Verification items for the finished model (mm, model axes). A direction names the side the tool comes from. Give positions to 0.01 mm unless a question says otherwise; leave off trailing zeros. Loops run counter-clockwise (first coordinate to the right, second up) from the corner with the lowest first, then second, coordinate; pieces in that order, holes last. Notation, with made-up numbers: M 66.5,69 L 89.5,69 A26 ccw 89.5,101 Z; hole C -27,-32 d10. An arc over 180 degrees is marked long. Write each question's results on one line, items separated by ' | '. Start each with the question number.
Autodesk Inventor part; units mm, degrees
ref_plane "YZ Plane" through (0, 0, 0) normal (1, 0, 0) x (0, 1, 0)
ref_plane "XZ Plane" through (0, 0, 0) normal (0, 1, 0) x (-1, 0, 0)
ref_plane "XY Plane" through (0, 0, 0) normal (0, 0, 1) x (1, 0, 0)
sketch "Sketch2" plane through (0, 0, 0) normal (0, 1, 0) x (-1, 0, 0)
  line L0 (35.4299, 28.2779) -> (35.4299, 34.5151)
  line L1 (35.4299, 51.0151) -> (35.4299, 60.0151)
  line L2 (47.4299, 49.0151) -> (37.4299, 49.0151)
  line L3 (20.9299, 49.0151) -> (12.9299, 49.0151)
  line L4 (22.9299, 55.7744) -> (22.9299, 51.0151)
  line L5 (22.9299, 34.5151) -> (22.9299, 26.5151)
  line L6 (12.9299, 36.5151) -> (20.9299, 36.5151)
  line L7 (37.4299, 36.5151) -> (47.4299, 36.5151)
  line L8 (12.9299, 38.5151) -> (14.9299, 38.5151)
  line L9 (14.9299, 38.5151) -> (14.9299, 40.0151)
  line L10 (14.9299, 40.0151) -> (12.9299, 40.0151)
  line L11 (12.9299, 42.0151) -> (14.9299, 42.0151)
  line L12 (14.9299, 42.0151) -> (14.9299, 43.5151)
  line L13 (14.9299, 43.5151) -> (12.9299, 43.5151)
  line L14 (12.9299, 45.5151) -> (14.9299, 45.5151)
  line L15 (14.9299, 45.5151) -> (14.9299, 47.0151)
  line L16 (14.9299, 47.0151) -> (12.9299, 47.0151)
  line L17 (12.9299, 49.0151) -> (12.9299, 47.0151)
  line L18 (12.9299, 45.5151) -> (12.9299, 43.5151)
  line L19 (12.9299, 42.0151) -> (12.9299, 40.0151)
  line L20 (12.9299, 38.5151) -> (12.9299, 36.5151)
  line L21 (33.4299, 27.5151) -> (33.4299, 25.5151)
  line L22 (31.9299, 25.5151) -> (31.9299, 27.5151)
  line L23 (29.9299, 27.5151) -> (29.9299, 25.5151)
  line L24 (28.4299, 25.5151) -> (28.4299, 27.5151)
  line L25 (26.4299, 27.5151) -> (26.4299, 25.5151)
  line L26 (24.9299, 25.5151) -> (24.9299, 27.5151)
  line L27 (47.4299, 47.0151) -> (45.4299, 47.0151)
  line L28 (47.4299, 45.5151) -> (45.4299, 45.5151)
  line L29 (47.4299, 43.5151) -> (45.4299, 43.5151)
  line L30 (47.4299, 42.0151) -> (45.4299, 42.0151)
  line L31 (47.4299, 40.0151) -> (45.4299, 40.0151)
  line L32 (47.4299, 38.5151) -> (45.4299, 38.5151)
  line L33 (45.4299, 38.5151) -> (45.4299, 40.0151)
  line L34 (45.4299, 42.0151) -> (45.4299, 43.5151)
  line L35 (45.4299, 45.5151) -> (45.4299, 47.0151)
  line L36 (47.4299, 36.5151) -> (47.4299, 38.5151)
  line L37 (47.4299, 40.0151) -> (47.4299, 42.0151)
  line L38 (47.4299, 43.5151) -> (47.4299, 45.5151)
  line L39 (47.4299, 47.0151) -> (47.4299, 49.0151)
  line L40 (33.4299, 60.0151) -> (33.4299, 58.0151)
  line L41 (31.9299, 60.0151) -> (31.9299, 58.0151)
  line L42 (29.9299, 60.0151) -> (29.9299, 58.0151)
  line L43 (28.4299, 60.0151) -> (28.4299, 58.0151)
  line L44 (26.4299, 60.0151) -> (26.4299, 58.0151)
  line L45 (24.9299, 60.0151) -> (24.9299, 58.0151)
  arc A0 (35.4299, 51.0151) -> (37.4299, 49.0151) centre (37.4299, 51.0151) ccw
  arc A1 (37.4299, 36.5151) -> (35.4299, 34.5151) centre (37.4299, 34.5151) ccw
  arc A2 (22.9299, 34.5151) -> (20.9299, 36.5151) centre (20.9299, 34.5151) ccw
  arc A3 (20.9299, 49.0151) -> (22.9299, 51.0151) centre (20.9299, 51.0151) ccw
  line L46 (35.4299, 28.2779) -> (35.4299, 25.5151)
  line L47 (22.9299, 26.5151) -> (22.9299, 25.5151)
  line L48 (35.4299, 25.5151) -> (33.4299, 25.5151)
  line L49 (31.9299, 25.5151) -> (29.9299, 25.5151)
  line L50 (28.4299, 25.5151) -> (26.4299, 25.5151)
  line L51 (24.9299, 25.5151) -> (22.9299, 25.5151)
  line L52 (24.9299, 27.5151) -> (26.4299, 27.5151)
  line L53 (28.4299, 27.5151) -> (29.9299, 27.5151)
  line L54 (31.9299, 27.5151) -> (33.4299, 27.5151)
  line L55 (22.9299, 55.7744) -> (22.9299, 60.0151)
  line L56 (35.4299, 60.0151) -> (33.4299, 60.0151)
  line L57 (31.9299, 60.0151) -> (29.9299, 60.0151)
  line L58 (28.4299, 60.0151) -> (26.4299, 60.0151)
  line L59 (24.9299, 60.0151) -> (22.9299, 60.0151)
  line L60 (24.9299, 58.0151) -> (26.4299, 58.0151)
  line L61 (28.4299, 58.0151) -> (29.9299, 58.0151)
  line L62 (31.9299, 58.0151) -> (33.4299, 58.0151)
  circle A4 centre (29.1799, 42.7651) radius 5.5
  point P0 (0, 0)
  point P1 (35.4299, 36.5151)
  point P2 (35.4299, 49.0151)
  point P3 (22.9299, 49.0151)
  point P4 (22.9299, 36.5151)
  dimension "d25" = 1.5
  dimension "d26" = 1.5
  dimension "d27" = 1.5
  dimension "d28" = 2
  dimension "d29" = 2
  dimension "d30" = 2
  dimension "d31" = 2
  dimension "d43" = 2
  dimension "d44" = 2
  dimension "d45" = 2
  dimension "d46" = 2
  dimension "d47" = 2
  dimension "d48" = 2
  dimension "d49" = 2
  dimension "d50" = 2
  dimension "d51" = 2
  dimension "d52" = 2
  dimension "d53" = 2
  dimension "d60" = 2
  dimension "d61" = 1.5
  dimension "d62" = 1.5
  dimension "d63" = 1.5
  dimension "d64" = 1.5
  dimension "d65" = 1.5
  dimension "d66" = 1.5
  dimension "d67" = 1.5
  dimension "d68" = 1.5
  dimension "d69" = 1.5
  dimension "d70" = 2
  dimension "d71" = 2
  dimension "d72" = 2
  dimension "d74" = 2
  dimension "d75" = 2
  dimension "d76" = 2
  dimension "d77" = 2
  dimension "d78" = 2
  dimension "d79" = 2
  dimension "d80" = 2
  dimension "d81" = 11
  dimension "d82" = 11
  dimension "d83" = 11
  dimension "d84" = 11
  dimension "d85" = 2
  dimension "d86" = 2
  dimension "d87" = 2
  dimension "d88" = 2
  dimension "d89" = 10
  dimension "d90" = 10
  dimension "d91" = 12
  dimension "d92" = 12
  dimension "d97" = 2
  dimension "d98" = 2
  dimension "d99" = 2
  dimension "d100" = 8
  dimension "d102" = 2
  dimension "d105" = 6.25
  dimension "d106" = 6.25
  dimension "d109" = 2
  dimension "d110" = 0
  dimension "d111" = 2
  dimension "d112" = 0
  dimension "d113" = 2
extrude "Extrusion3" add sketch "Sketch2" along normal blind 1.524
properties part number "cross"
1. Set-up check for faces 4 (the face through (-14, 1, 38.515)), 5 (the face through (-46, 1, 38.515)), 6 (the face through (-26, 1, 27.515)), 7 (the face through (-31.93, 1, 59)): record each of +Z, -Z, +X, -X, +Y, -Y from which the full face is reachable in a straight line by a thin tool's end or side.
2. Release check for a two-part mould opening along Z. For faces 1 (the face through (-27, 1, 25.515)), 2 (the face through (-17, 1, 49.015)), 3 (the face through (-14.93, 1, 43)) record: released by +Z, released by -Z, zero draft, split by the parting line, or undercut.
3. Depth check by flat-ended pin: pin 1 Ø0.8 at (x, y) = (-29, 0.5) entering from -Z; pin 2 Ø0.8 at (y, z) = (0.5, 26) entering from +X; pin 3 Ø3 at (x, z) = (-41, 46) entering from -Y; pin 4 Ø0.8 at (y, z) = (0.5, 26.5) entering from -X. Enter the tip coordinate at first touch or a pass-through.
4. Section check C-C, the plane x = -39.5. Record the boundary of the cut face in (y, z).
5. Thickness scan on probe 1 along X at (y, z) = (0.35, 38); probe 2 along Z at (x, y) = (-19.5, 0.1); probe 3 along X at (y, z) = (0.8, 41). Record the ranges inside material, lowest first.
6. Section check B-B, the plane x = -29. Record the boundary of the cut face in (y, z), plus the area to 3 significant figures.
7. Section check D-D, the plane z = 56. Record the boundary of the cut face in (x, y), plus the area to 4 significant figures.
8. Section check A-A, the plane z = 41.5. Record the boundary of the cut face in (x, y).
Filled sheet:
1) face 4: +X, +Y, -Y | face 5: -X, +Y, -Y | face 6: -Z, +Y, -Y | face 7: +Z, +Y, -Y
2) face 1: released by -Z | face 2: released by +Z | face 3: undercut
3) pin 1: z = 27.52 | pin 2: x = -22.93 | pin 3: y = 0 | pin 4: x = -35.43
4) outline: M 0,36.52 L 1.52,36.52 L 1.52,49.02 L 0,49.02 Z
5) probe 1: -47.43 to -31.93, -26.43 to -12.93 | probe 2: 36.52 to 49.02 | probe 3: -47.43 to -34.39, -23.97 to -12.93
6) outline: M 0,27.52 L 1.52,27.52 L 1.52,37.27 L 0,37.27 Z; M 0,48.26 L 1.52,48.26 L 1.52,58.02 L 0,58.02 Z | area: 29.7 mm2
7) outline: M -35.43,0 L -22.93,0 L -22.93,1.52 L -35.43,1.52 Z | area: 19.05 mm2
8) outline: M -47.43,0 L -34.53,0 L -34.53,1.52 L -47.43,1.52 Z; M -23.83,0 L -12.93,0 L -12.93,1.52 L -23.83,1.52 Z
